Verification items for this drawing (mm, ordinates from the low corner). A direction names the side the tool comes from. Coordinates: 2 decimals unless noted, no trailing zeros. Loops run counter-clockwise (first coordinate to the right, second up) from the corner with the lowest first, then second, coordinate; pieces in that order, holes last. Notation, with made-up numbers: (80, 30) - (96, 30) arc R23 ccw to (96, 44) - close; hole circle Ø5 at (15, 66.25). An arc over 180 degrees is marked (long way). One line per item, written item: value. Start each with the question number.
(1) Set-up check for the marked faces 4, 5, 6 and 7: record each of +Z, -Z, +X, -X, +Y, -Y from which the full face is reachable in a straight line by a thin tool's end or side.
(2) Section check B-B (z = 35.5). Record the boundary of the cut face in (x, y).
(3) Gauge pin test, flat ends, axial feed: P1, Ø7.5, axis at x = 22, y = 7.5, coming from the +Z side; P2, Ø6, axis at x = 17, z = 24, coming from the +Y side (1 decimal); P3, Ø20, axis at y = 11, z = 20, coming from the +X side. Record the tip position at first contact, or that the pin passes through.
(4) Thickness scan on probe 1 along Y at (x, z) = (32, 20); probe 2 along Z at (x, y) = (31.5, 145); probe 3 along X at (y, z) = (18, 28). Record the ranges inside material, lowest first. Write a range as [from, to].
(5) Section check D-D (z = 7.5). Record the boundary of the cut face in (x, y) (1 decimal).
(6) Draft check along Z on the marked faces 1, 2 and 3. Enter one of: +Z half, -Z half, draft (parallel to the pull), parting line (faces both ways), or undercut.
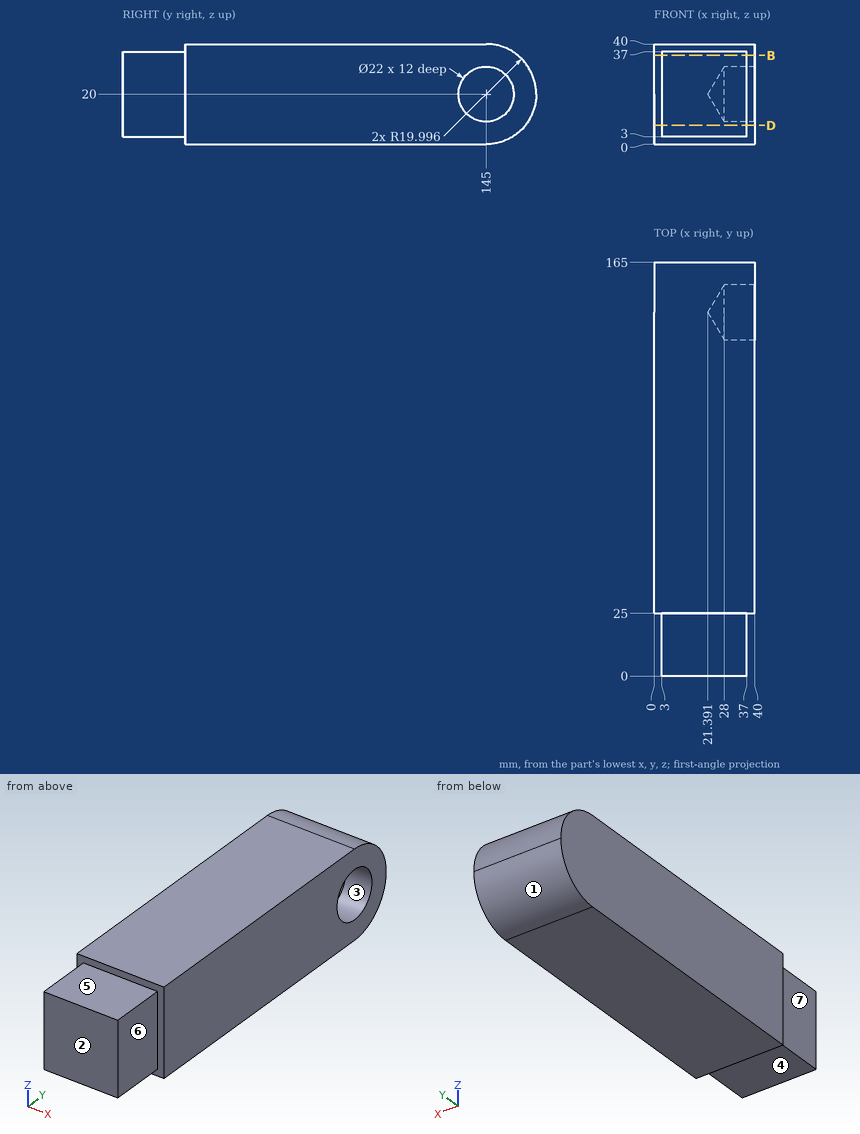
Responses:
1. face 4: -Z, +X, -X, -Y
1. face 5: +Z, +X, -X, -Y
1. face 6: +Z, -Z, +X, -Y
1. face 7: +Z, -Z, -X, -Y
2. outline: (0, 25) - (3, 25) - (3, 0) - (37, 0) - (37, 25) - (40, 25) - (40, 157.64) - (0, 157.64) - close
3. P1: stops at z = 37
3. P2: stops at y = 165
3. P3: stops at x = 37
4. probe 1: y = [0, 134], [156, 165]
4. probe 2: z = [0, 9], [31, 40]
4. probe 3: x = [3, 37]
5. outline: (0, 25) - (3, 25) - (3, 0) - (37, 0) - (37, 25) - (40, 25) - (40, 160.6) - (0, 160.6) - close
6. face 1: -Z half
6. face 2: draft
6. face 3: undercut
